Could you check a few things on this model? Use its own coordinates, in mm. A direction names the side the tool comes from. Give positions to 0.01 mm unless a question says otherwise; leave off trailing zeros. Order: outer loops, then holes, each group sorted by start corner. A loop starts at its lowest first (then second) coordinate and runs counter-clockwise, first axis right, second up. Notation, with made-up numbers: (14, 34) -> (38, 34) arc R18 ccw to (38, 62) -> close; hole circle Ø9 at (45.5, -20). An arc over 180 degrees is marked (long way). Write each question's results on one line, items separated by ' | '.
```python
from build123d import *

# Parameters (mm, degrees)
SKETCH1_W           = 40.05
SKETCH1_H           = 20
SKETCH1_R           = 7.5
SKETCH1_R_2         = 3
BOSS_EXTRUDE1_DEPTH = 40
BOSS_EXTRUDE2_START = -6.75
SKETCH1_3_W         = 7.4
SKETCH1_3_H         = 17.9
SKETCH1_3_R         = 2.15
BOSS_EXTRUDE2_DEPTH = 2.6
SKETCH1_4_R         = 7.5
SKETCH1_4_R_2       = 3
BOSS_EXTRUDE3_DEPTH = 4.4
BOSS_EXTRUDE4_START = 4.4
SKETCH1_5_R         = 3
BOSS_EXTRUDE4_DEPTH = 4.1
FILLET1_R           = 0.5


with BuildPart() as part:
    # Sketch1 → Boss-Extrude1 (new body)
    # profile 1 of 3: a face of its own
    with BuildSketch(Plane(origin=(0, 0, 0), x_dir=(1, 0, 0), z_dir=(0, 1, 0))):
        Rectangle(SKETCH1_W, SKETCH1_H)
        with Locations((-10.025, 0)):
            Circle(SKETCH1_R, mode=Mode.SUBTRACT)
    # profile 2 of 3: a face of its own
    with BuildSketch(Plane(origin=(0, 0, 0), x_dir=(1, 0, 0), z_dir=(0, 1, 0))):
        with Locations((-10.025, 0)):
            Circle(SKETCH1_R)
        with Locations((-10.025, 0)):
            Circle(SKETCH1_R_2, mode=Mode.SUBTRACT)
    # profile 3 of 3: a face of its own
    with BuildSketch(Plane(origin=(0, 0, 0), x_dir=(1, 0, 0), z_dir=(0, 1, 0))):
        with Locations((-10.025, 0)):
            Circle(SKETCH1_R_2)
    extrude(amount=-BOSS_EXTRUDE1_DEPTH)

    # Sketch1<3> → Boss-Extrude2 (add)
    # profile 1 of 2: a face of its own
    with BuildSketch(Plane(origin=(0, 0, 0), x_dir=(1, 0, 0), z_dir=(0, 1, 0)).offset(BOSS_EXTRUDE2_START)):
        with Locations((-23.725, 0)):
            Rectangle(SKETCH1_3_W, SKETCH1_3_H)
        with Locations(Location((-23.725, -5, 0), (0, 0, 270))):
            Circle(SKETCH1_3_R, mode=Mode.SUBTRACT)
        with Locations(Location((-23.725, 5, 0), (0, 0, 270))):
            Circle(SKETCH1_3_R, mode=Mode.SUBTRACT)
    # profile 2 of 2: a face of its own
    with BuildSketch(Plane(origin=(0, 0, 0), x_dir=(1, 0, 0), z_dir=(0, 1, 0)).offset(BOSS_EXTRUDE2_START)):
        with Locations((23.725, 0)):
            Rectangle(SKETCH1_3_W, SKETCH1_3_H)
        with Locations(Location((23.725, -5, 0), (0, 0, 270))):
            Circle(SKETCH1_3_R, mode=Mode.SUBTRACT)
        with Locations(Location((23.725, 5, 0), (0, 0, 270))):
            Circle(SKETCH1_3_R, mode=Mode.SUBTRACT)
    extrude(amount=-BOSS_EXTRUDE2_DEPTH)

    # Sketch1<4> → Boss-Extrude3 (add)
    # profile 1 of 2: a face of its own
    with BuildSketch(Plane(origin=(0, 0, 0), x_dir=(1, 0, 0), z_dir=(0, 1, 0))):
        with Locations(Location((-10.025, 0, 0), (0, 0, 270))):
            Circle(SKETCH1_4_R)
        with Locations((-10.025, 0)):
            Circle(SKETCH1_4_R_2, mode=Mode.SUBTRACT)
    # profile 2 of 2: a face of its own
    with BuildSketch(Plane(origin=(0, 0, 0), x_dir=(1, 0, 0), z_dir=(0, 1, 0))):
        with Locations((-10.025, 0)):
            Circle(SKETCH1_4_R_2)
    extrude(amount=BOSS_EXTRUDE3_DEPTH)

    # Sketch1<5> → Boss-Extrude4 (add)
    with BuildSketch(Plane(origin=(0, 0, 0), x_dir=(1, 0, 0), z_dir=(0, 1, 0)).offset(BOSS_EXTRUDE4_START)):
        with Locations(Location((-10.025, 0, 0), (0, 0, 270))):
            Circle(SKETCH1_5_R)
    extrude(amount=BOSS_EXTRUDE4_DEPTH)

    # Fillet1
    fillet1_edges = [part.edges().sort_by_distance(p)[0] for p in [
        (20.025, -40, 0),
        (0, -40, -10),
        (-27.425, -6.75, 0),
        (-27.425, -8.05, 8.95),
        (-23.725, -9.35, -8.95),
        (-27.425, -8.05, -8.95),
        (-23.725, -6.75, 8.95),
        (-20.025, -40, 0),
        (-27.425, -9.35, 0),
        (-23.725, -9.35, 8.95),
        (-23.725, -6.75, -8.95),
        (23.725, -6.75, -8.95),
        (27.425, -9.35, 0),
        (27.425, -8.05, -8.95),
        (23.725, -9.35, 8.95),
        (27.425, -8.05, 8.95),
        (23.725, -9.35, -8.95),
        (23.725, -6.75, 8.95),
        (27.425, -6.75, 0),
        (0, -40, 10),
        (-10.025, 4.4, -7.5),
        (-10.025, 8.5, -3),
        (-20.025, 0, 0),
        (0, 0, -10),
        (20.025, 0, 0),
        (0, 0, 10),
        (-20.025, -20, 10),
        (-20.025, -20, -10),
        (20.025, -20, -10),
        (20.025, -20, 10),
    ]]
    fillet(fillet1_edges, radius=FILLET1_R)


solid = part.part
```
Q1. Suppose I cut it at C-C on y = -19. Please give me the cut outline in (x, z) (3 decimals).
Here are the results:
outline: (-20.025, -9.5) arc R0.5 ccw to (-19.525, -10) -> (19.525, -10) arc R0.5 ccw to (20.025, -9.5) -> (20.025, 9.5) arc R0.5 ccw to (19.525, 10) -> (-19.525, 10) arc R0.5 ccw to (-20.025, 9.5) -> close
Q2. Thinking about a two-plate mould opening in X: for faces 5 (the cylindrical face through (25.857, -8.032, 4.72)), 6 (the flat face through (-27.425, -8, 0)), 7 (the flat face through (0, -20, 10)), 8 (the cylindrical face through (-9.695, 1.923, -7.493)), which applies, +X half, -X half, draft (parallel to the pull), parting line (faces both ways), or undercut?
Here are the results:
face 5: undercut | face 6: -X half | face 7: draft | face 8: parting line
Q3. I need wall thicknesses on line 1 along X through (y, z) = (-8.35, -5) (3 decimals); line 2 along X through (y, z) = (-8.5, 4.25) (3 decimals); line 3 along Y through (x, z) = (1.5, -7.5). Which ranges of each line are inside material? Lowest first, please.
Here are the results:
line 1: x = -27.425 to -25.875, -21.575 to 21.575, 25.875 to 27.425 | line 2: x = -27.425 to -25.74, -21.71 to 21.71, 25.74 to 27.425 | line 3: y = -40 to 0
Q4. I'm going to push flat-ended pins straight in: pin 1 Ø5.5 at (x, z) = (-23.5, -4) entering from +Y; pin 2 Ø2 at (y, z) = (-17, 7) entering from -X (3 decimals); pin 3 Ø8 at (x, y) = (3.5, 2) entering from -Z; pin 4 Ø1.8 at (x, y) = (23.5, -8) entering from +Z. Where does each tip first touch, or does it pass through?
Here are the results:
pin 1: stops at y = -6.75 | pin 2: stops at x = -20.025 | pin 3: stops at z = -10 | pin 4: stops at z = 8.95
Q5. Suppose I cut it at A-A on x = 13.5. Please give me the cut outline in (y, z), and give its area (3 significant figures).
Here are the results:
outline: (-40, -9.5) arc R0.5 ccw to (-39.5, -10) -> (-0.5, -10) arc R0.5 ccw to (0, -9.5) -> (0, 9.5) arc R0.5 ccw to (-0.5, 10) -> (-39.5, 10) arc R0.5 ccw to (-40, 9.5) -> close | area: 800 mm²
Q6. Suppose I cut it at D-D on z = -5. State how many separate pieces and enclosed holes the cut face has, and give its area (3 significant figures).
Here are the results:
separate pieces: 3 | enclosed holes: 0 | area: 1,670 mm²
Q7. For faces 1 (the flat face through (23, -8, -8.95)), 2 (the flat face through (-13, 4.4, 1.5)), 3 (the flat face through (23, -6.75, 0)), 4 (the flat face through (23, -8, 8.95)), which set-ups out of +Z, -Z, +X, -X, +Y, -Y let a thin tool reach every point of the face, with its end or its side?
Here are the results:
face 1: -Z, +X, +Y, -Y | face 2: +Y | face 3: +Z, -Z, +X, +Y | face 4: +Z, +X, +Y, -Y
